For this review, take the finished solid that the model builds, in its own axes (mm). A direction names the side the tool comes from. Round coordinates to 2 decimals unless told otherwise and drop trailing zeros.
1) Tool access review of faces 1 (the flat face through (-3.08, 17.3, 14.56)), 2 (the flat face through (-20, 17, 8)): name each direction out of +Z, -Z, +X, -X, +Y, -Y from which nothing blocks a thin tool from reaching the whole face with its end or side.
2) Mouldability with a two-part tool opening along Y and no side actions: class faces 3 (the flat face through (-10, 34, 8)), 4 (the flat face through (-9.712, 17, 15)), 5 (the flat face through (-12, 17, 15.3)) as pulls with the +Y half, pulls with the -Y half, needs draft (parallel to the pull), parting line crosses it, or undercut.
3) Insertion check: pin 1 (4 mm diameter, centred on x = -17, z = 13, fed in from -Y). The pin has a flat end and moves straight along its axis. Give the tip position at first contact, or say it passes through.
```python
from build123d import *

# Parameters (mm, degrees)
ESBO_O1_W                = 20
ESBO_O1_H                = 34
RESSALTO_EXTRUS_O1_DEPTH = 15.3
ESBO_O2_W                = 0.628205129
ESBO_O2_H                = 2.557692308
ESBO_O2_W_2              = 1.211538461
ESBO_O2_H_2              = 0.583333334
ESBO_O2_W_3              = 0.628205128
CORTE_EXTRUS_O1_DEPTH    = 1.5


with BuildPart() as part:
    # Esboço1 → Ressalto-extrusão1 (new body)
    with BuildSketch(Plane.XY):
        with Locations((-10, 17)):
            Rectangle(ESBO_O1_W, ESBO_O1_H)
    extrude(amount=RESSALTO_EXTRUS_O1_DEPTH)

    # Esboço2 → Corte-extrusão1 (cut)
    with BuildSketch(Plane.XY.offset(15.3)):
        Polygon((-16.80198257, 18.779052447), (-16.173777441, 18.779052447), (-16.173777441, 17.432898601), (-14.96223898, 17.432898601), (-14.96223898, 18.779052447), (-14.334033852, 18.779052447), (-14.334033852, 15.279052447), (-14.96223898, 15.279052447), (-14.96223898, 16.804693473), (-16.173777441, 16.804693473), (-16.173777441, 15.279052447), (-16.80198257, 15.279052447), align=None)
        with BuildLine():
            add(Edge.make_bspline(
                [(-13.348256608, 18.913667832), (-13.321180971, 18.912339399), (-13.26801535, 18.909730892), (-13.191848363, 18.884303755), (-13.121942506, 18.844396624), (-13.060143789, 18.789643089), (-13.008745395, 18.724257353), (-12.969475113, 18.651053675), (-12.947599275, 18.569946357), (-12.944561045, 18.51391827), (-12.943008211, 18.485282415)],
                knots=[0, 0, 0, 0, 0.989868614, 1.943702388, 2.910836514, 3.924849579, 4.949916355, 5.946401046, 6.950409252, 8, 8, 8, 8], degree=3))
            add(Edge.make_bspline(
                [(-12.943008211, 18.485282415), (-12.944505487, 18.456857591), (-12.947423001, 18.401470467), (-12.969978599, 18.321464218), (-13.007672708, 18.248296095), (-13.059487397, 18.183881459), (-13.120616135, 18.130009762), (-13.188994496, 18.089378141), (-13.264431582, 18.06536551), (-13.316772234, 18.062538947), (-13.343348756, 18.061103729)],
                knots=[0, 0, 0, 0, 1.05296456, 2.051751585, 3.055639087, 4.085634717, 5.099016424, 6.062201612, 7.016062274, 8, 8, 8, 8], degree=3))
            add(Edge.make_bspline(
                [(-13.343348756, 18.061103729), (-13.37066074, 18.062427414), (-13.4242889, 18.06502652), (-13.501080613, 18.09051315), (-13.571918836, 18.130105987), (-13.63344947, 18.185978222), (-13.685436491, 18.251828573), (-13.722991431, 18.326736496), (-13.746482976, 18.408398424), (-13.749271401, 18.465256325), (-13.750700518, 18.494396998)],
                knots=[0, 0, 0, 0, 0.989065327, 1.942068821, 2.907541208, 3.917690034, 4.939857478, 5.938239964, 6.943311734, 8, 8, 8, 8], degree=3))
            add(Edge.make_bspline(
                [(-13.750700518, 18.494396998), (-13.749145248, 18.522339152), (-13.746090144, 18.57722748), (-13.724083268, 18.656531545), (-13.685713452, 18.728504555), (-13.634685286, 18.792693343), (-13.57342937, 18.846425519), (-13.503565478, 18.885120645), (-13.427911097, 18.909497568), (-13.375082261, 18.912263391), (-13.348256608, 18.913667832)],
                knots=[0, 0, 0, 0, 1.038616768, 2.040212704, 3.031499824, 4.052181184, 5.074969369, 6.039807101, 7.004644834, 8, 8, 8, 8], degree=3))
        make_face()
        with Locations((-13.346854365, 16.557898601)):
            Rectangle(ESBO_O2_W, ESBO_O2_H)
        with Locations((-11.753905647, 16.557898601)):
            Rectangle(ESBO_O2_W_2, ESBO_O2_H_2)
        Polygon((-10.340444108, 18.779052447), (-9.71223898, 18.779052447), (-9.71223898, 15.907257575), (-8.725059493, 15.907257575), (-8.725059493, 15.279052447), (-10.340444108, 15.279052447), align=None)
        with BuildLine():
            add(Edge.make_bspline(
                [(-8.008513018, 18.913667832), (-7.981437382, 18.912339399), (-7.928271761, 18.909730892), (-7.852104774, 18.884303755), (-7.782198916, 18.844396624), (-7.720400199, 18.789643089), (-7.669001805, 18.724257353), (-7.629731523, 18.651053675), (-7.607855685, 18.569946357), (-7.604817455, 18.51391827), (-7.603264621, 18.485282415)],
                knots=[0, 0, 0, 0, 0.989868614, 1.943702388, 2.910836514, 3.924849579, 4.949916355, 5.946401046, 6.950409252, 8, 8, 8, 8], degree=3))
            add(Edge.make_bspline(
                [(-7.603264621, 18.485282415), (-7.604761897, 18.456857591), (-7.607679411, 18.401470467), (-7.630235009, 18.321464218), (-7.667929118, 18.248296095), (-7.719743807, 18.183881459), (-7.780872545, 18.130009762), (-7.849250906, 18.089378141), (-7.924687993, 18.06536551), (-7.977028644, 18.062538947), (-8.003605166, 18.061103729)],
                knots=[0, 0, 0, 0, 1.05296456, 2.051751585, 3.055639087, 4.085634717, 5.099016424, 6.062201612, 7.016062274, 8, 8, 8, 8], degree=3))
            add(Edge.make_bspline(
                [(-8.003605166, 18.061103729), (-8.03091715, 18.062427414), (-8.08454531, 18.06502652), (-8.161337023, 18.09051315), (-8.232175246, 18.130105987), (-8.293705881, 18.185978222), (-8.345692901, 18.251828573), (-8.383247842, 18.326736496), (-8.406739386, 18.408398424), (-8.409527811, 18.465256325), (-8.410956929, 18.494396998)],
                knots=[0, 0, 0, 0, 0.989065327, 1.942068821, 2.907541208, 3.917690034, 4.939857478, 5.938239964, 6.943311734, 8, 8, 8, 8], degree=3))
            add(Edge.make_bspline(
                [(-8.410956929, 18.494396998), (-8.409401658, 18.522339152), (-8.406346555, 18.57722748), (-8.384339678, 18.656531545), (-8.345969862, 18.728504555), (-8.294941696, 18.792693343), (-8.23368578, 18.846425519), (-8.163821888, 18.885120645), (-8.088167507, 18.909497568), (-8.035338671, 18.912263391), (-8.008513018, 18.913667832)],
                knots=[0, 0, 0, 0, 1.038616768, 2.040212704, 3.031499824, 4.052181184, 5.074969369, 6.039807101, 7.004644834, 8, 8, 8, 8], degree=3))
        make_face()
        with Locations((-8.007110775, 16.557898601)):
            Rectangle(ESBO_O2_W_3, ESBO_O2_H)
        with BuildLine():
            Line((-7.109674877, 17.836744755), (-6.481469749, 17.836744755))
            Line((-6.481469749, 17.836744755), (-6.481469749, 17.566111742))
            add(Edge.make_bspline(
                [(-6.481469749, 17.566111742), (-6.445630958, 17.593987892), (-6.377136061, 17.647264633), (-6.273011992, 17.71519275), (-6.174731762, 17.770789186), (-6.0801046, 17.81307868), (-5.987350094, 17.843504153), (-5.894966016, 17.86536304), (-5.801576583, 17.879359886), (-5.738796215, 17.880864732), (-5.707431288, 17.88161655)],
                knots=[0, 0, 0, 0, 1.276643801, 2.439914479, 3.493451431, 4.44993799, 5.350072675, 6.235028322, 7.118224225, 8, 8, 8, 8], degree=3))
            add(Edge.make_bspline(
                [(-5.707431288, 17.88161655), (-5.67561579, 17.880757378), (-5.613159296, 17.879070751), (-5.52119555, 17.867274166), (-5.433333122, 17.845788847), (-5.348584071, 17.817262154), (-5.267810997, 17.779608556), (-5.190024382, 17.734901017), (-5.116895054, 17.68044421), (-5.071858776, 17.638972521), (-5.049077922, 17.617994755)],
                knots=[0, 0, 0, 0, 1.048836932, 2.058954983, 3.049370783, 4.026390553, 5.001981509, 5.982488534, 6.97947532, 8, 8, 8, 8], degree=3))
            add(Edge.make_bspline(
                [(-5.049077922, 17.617994755), (-5.030806839, 17.5985545), (-4.99413095, 17.559531712), (-4.947978953, 17.492753726), (-4.908375347, 17.419953499), (-4.875925695, 17.340291256), (-4.85194671, 17.253329305), (-4.83349935, 17.160118021), (-4.823148214, 17.060135491), (-4.821870317, 16.991448437), (-4.821213339, 16.956135781)],
                knots=[0, 0, 0, 0, 0.889584746, 1.785680191, 2.700364693, 3.65222533, 4.649950538, 5.707241244, 6.821271309, 8, 8, 8, 8], degree=3))
            Line((-4.821213339, 16.956135781), (-4.821213339, 15.279052447))
            Line((-4.821213339, 15.279052447), (-5.449418467, 15.279052447))
            Line((-5.449418467, 15.279052447), (-5.449418467, 16.38962937))
            add(Edge.make_bspline(
                [(-5.449418467, 16.38962937), (-5.449551319, 16.425854455), (-5.449805904, 16.495273106), (-5.451760555, 16.594621628), (-5.455577174, 16.684346245), (-5.459055922, 16.764610319), (-5.465886088, 16.83512886), (-5.472045642, 16.896348304), (-5.48149688, 16.947713262), (-5.493794475, 17.002963982), (-5.515269103, 17.062119982), (-5.548607417, 17.1244506), (-5.590901743, 17.17740185), (-5.640424613, 17.221344946), (-5.697121331, 17.256107965), (-5.760306801, 17.280565915), (-5.829642274, 17.295808709), (-5.877954417, 17.297437394), (-5.903044268, 17.298283216)],
                knots=[0, 0, 0, 0, 1.49886392, 2.872294502, 4.110984203, 5.214877267, 6.195405875, 7.042225351, 7.75923308, 8.355011229, 9.382752534, 10.352059385, 11.267231453, 12.171456522, 13.078624015, 14.003401117, 14.963110155, 16, 16, 16, 16], degree=3))
            add(Edge.make_bspline(
                [(-5.903044268, 17.298283216), (-5.935674676, 17.29662852), (-5.999506096, 17.293391611), (-6.091825477, 17.268982369), (-6.176619289, 17.227469432), (-6.253194699, 17.170023876), (-6.320822389, 17.099100218), (-6.376522348, 17.01451562), (-6.422207758, 16.918311526), (-6.441853163, 16.848066911), (-6.452022634, 16.811704691)],
                knots=[0, 0, 0, 0, 0.984188326, 1.925263693, 2.85911992, 3.81709677, 4.80007086, 5.801799564, 6.862098548, 8, 8, 8, 8], degree=3))
            add(Edge.make_bspline(
                [(-6.452022634, 16.811704691), (-6.454550151, 16.800284892), (-6.460187023, 16.774816444), (-6.464822638, 16.731790285), (-6.471271114, 16.680743913), (-6.473687199, 16.620753533), (-6.477888506, 16.552103054), (-6.47944235, 16.474701653), (-6.480998974, 16.388701101), (-6.481307625, 16.328632983), (-6.481469749, 16.297081293)],
                knots=[0, 0, 0, 0, 0.543362196, 1.211806945, 2.009705693, 2.934833164, 4.000995085, 5.207458376, 6.533175157, 8, 8, 8, 8], degree=3))
            Line((-6.481469749, 16.297081293), (-6.481469749, 15.279052447))
            Line((-6.481469749, 15.279052447), (-7.109674877, 15.279052447))
            Line((-7.109674877, 15.279052447), (-7.109674877, 17.836744755))
        make_face()
        Polygon((-4.193008211, 18.868796037), (-3.564803082, 18.868796037), (-3.564803082, 16.775246357), (-2.5874393, 17.836744755), (-1.811297473, 17.836744755), (-2.933793467, 16.617493954), (-1.650740582, 15.279052447), (-2.441605967, 15.279052447), (-3.564803082, 16.450626966), (-3.564803082, 15.279052447), (-4.193008211, 15.279052447), align=None)
    extrude(amount=-CORTE_EXTRUS_O1_DEPTH, mode=Mode.SUBTRACT)


solid = part.part
```
Response:
1. face 1: +Z
1. face 2: +Z, -Z, -X, +Y, -Y
2. face 3: pulls with the +Y half
2. face 4: undercut
2. face 5: needs draft
3. pin 1: stops at y = 0
